Study the drawing (mm; zero at the part's minimum x, y, z) and answer. Coordinates: 2 decimals unless noted, no trailing zeros. Order: outer loops, then holes, each group sorted by start corner. A loop starts at its lowest first (then second) coordinate and runs counter-clockwise, first axis right, second up. Notation, with made-up numbers: (35, 38) - (75, 38) arc R31 cw to (75, 74) - close; hole circle Ø6 at (8.25, 86). An arc over 180 degrees is marked (long way). Write item = value, one per line.
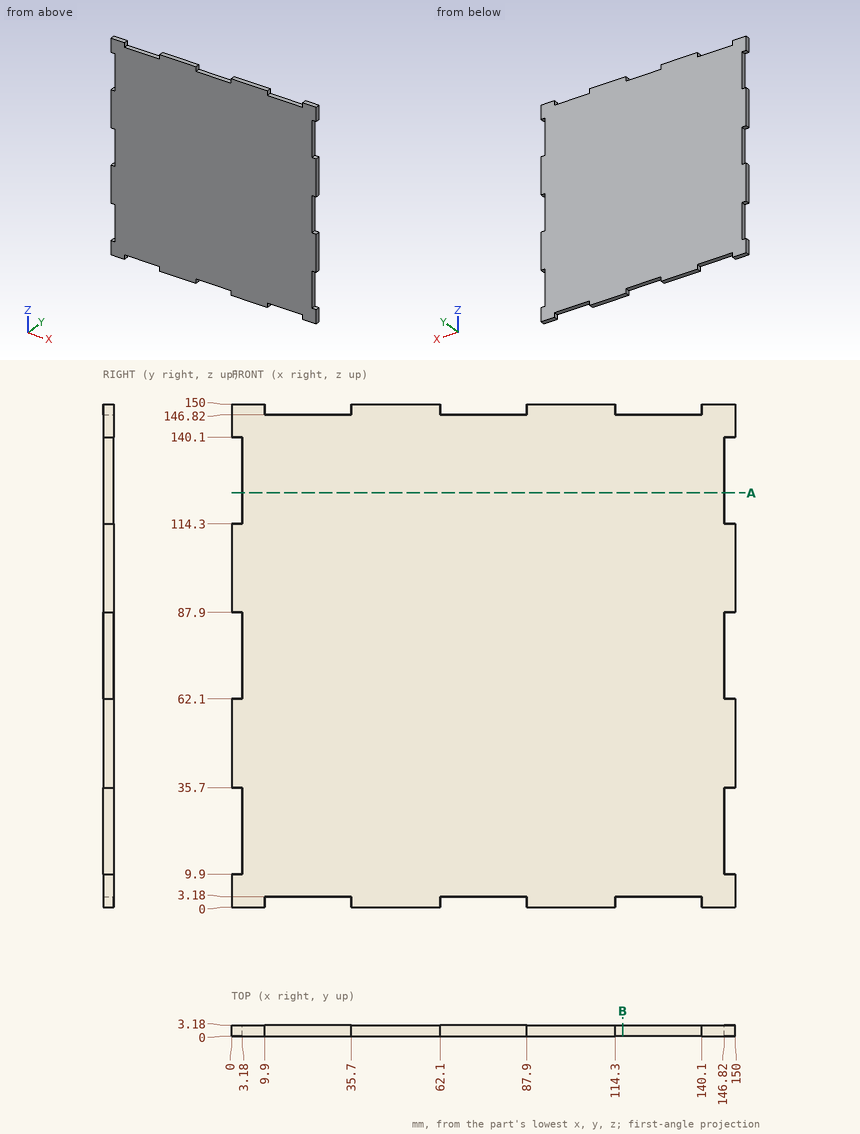
1) The part is cut by section A-A (z = 123.5). Determine the outline of the cut face in (x, y), and give its area (3 significant figures).
Returned:
outline = (3.18, 0) - (146.82, 0) - (146.82, 3.18) - (3.18, 3.18) - close
area = 457 mm^2
2) The part is cut by section B-B (x = 116.5). Determine the outline of the cut face in (y, z), and give its area (3 significant figures).
Returned:
outline = (0, 3.18) - (3.18, 3.18) - (3.18, 146.82) - (0, 146.82) - close
area = 457 mm^2
3) A straight line is drawn through the part: line 1 along Z through (x, y) = (17, 0.3). Find the intervals that lie inside material, in ascending order. Write a range as from..to.
Returned:
line_1 = 3.18..146.82
4) Flat-ended cylindrical pins translate along their axes: pin 1 Ø1 at (x, y) = (122, 1) entering from +Z; pin 2 Ø1.6 at (y, z) = (1.5, 71) entering from -X. Find the tip coordinate at first contact, or state that the pin passes through.
Returned:
pin_1 = 146.82
pin_2 = 3.18
